Can you work these out from the model? Positions are in its coordinate system, mm. Round coordinates to 2 decimals unless told otherwise and drop trailing zeros. Order: outer loops, then holes, each group sorted by start corner. A loop starts at its lowest first (then second) coordinate and runs counter-clockwise, first axis right, second up. Notation, with made-up numbers: (63.5, 12.5) - (80.5, 12.5) arc R6 cw to (80.5, 16.5) - close; hole circle Ø8 at (29, 86.25). An arc over 180 degrees is marked (long way). Write item = value, one per line.
from build123d import *

# Parameters (mm, degrees)
ESQUISSE1_R                     = 1.5
BOSS_EXTRU_1_DEPTH              = 4
ESQUISSE2_R                     = 2.95
BOSS_EXTRU_2_DEPTH              = 2.4
CHANFREIN1_SIZE                 = 2.2
ESQUISSE4_W                     = 0.2
ESQUISSE4_H                     = 5.9
ESQUISSE4_W_2                   = 5.9
ESQUISSE4_H_2                   = 0.2
ENL_V_DE_MAT_EXTRU_MINCE1_DEPTH = 0.2


with BuildPart() as part:
    # Esquisse1 → Boss.-Extru.1 (new body)
    with BuildSketch(Plane.XY):
        Circle(ESQUISSE1_R)
    extrude(amount=BOSS_EXTRU_1_DEPTH)

    # Esquisse2 → Boss.-Extru.2 (add)
    with BuildSketch(Plane(origin=(0, 0, 0), x_dir=(-1, 0, 0), z_dir=(0, 0, -1))):
        Circle(ESQUISSE2_R)
    extrude(amount=BOSS_EXTRU_2_DEPTH)

    # Chanfrein1
    # the kernel refuses this chamfer: 2.2 mm, written as the material it takes off along each edge
    with BuildSketch(Plane(origin=(0, 0, 0), x_dir=(-1, 0, 0), z_dir=(0, -1, 0))) as chanfrein1_piece_1_section:
        Polygon((2.95, CHANFREIN1_SIZE), (2.95 - CHANFREIN1_SIZE, 0), (2.95, 0), align=None)
    chanfrein1_piece_1 = revolve(axis=Axis((0, 0, 0), (0, 0, -1)), mode=Mode.PRIVATE)
    chanfrein1_piece_1 = chanfrein1_piece_1 - Plane(origin=(0, 0, -1.483070645), x_dir=(1, 0, 0), z_dir=(0, 0, -1)) * Cylinder(1.5, 12, mode=Mode.PRIVATE)
    add(chanfrein1_piece_1, mode=Mode.SUBTRACT)

    # Esquisse4 → Enlèv. de mat.-Extru.-Mince1 (cut)
    with BuildSketch(Plane(origin=(0, 0, -2.4), x_dir=(-1, 0, 0), z_dir=(0, 0, -1))):
        with Locations((-0.1, 0)):
            Rectangle(ESQUISSE4_W, ESQUISSE4_H)
        with Locations((0, -0.1)):
            Rectangle(ESQUISSE4_W_2, ESQUISSE4_H_2)
    extrude(amount=-ENL_V_DE_MAT_EXTRU_MINCE1_DEPTH, mode=Mode.SUBTRACT)


solid = part.part
(1) If I drill on line 1 (Y direction, x = -0.6, z = 2.75); line 2 (X direction, y = -2.3, z = -2); line 3 (Z direction, x = 2.45, y = 0.55), over which ranges is the centre line in solid material (lowest first)? Write a range as from..to.
Computed:
line_1 = -1.37..1.37
line_2 = -1.51..1.51
line_3 = -2.4..-1.76
(2) Thinking about a two-plate mould opening in Y: for faces 1 (the face through (-0.325, 1.464, 1.592)), 2 (the face through (-1, -1, -2.4)), which applies, +Y half, -Y half, draft (parallel to the pull), parting line (faces both ways), or undercut?
Computed:
face_1 = parting line
face_2 = draft
(3) If we section it at A-A (z = -1.5): Write out the boundary of the cut face in (x, y), plus the area to 3 significant figures.
Computed:
outline = circle Ø4.5 at (0, 0)
area = 15.9 mm^2
(4) Will this pin go through, and if not, where does the flat tip stop? P1, Ø1.5, axis at x = -0.5, z = 2, coming from the +Y side.
Computed:
P1 = 1.5
